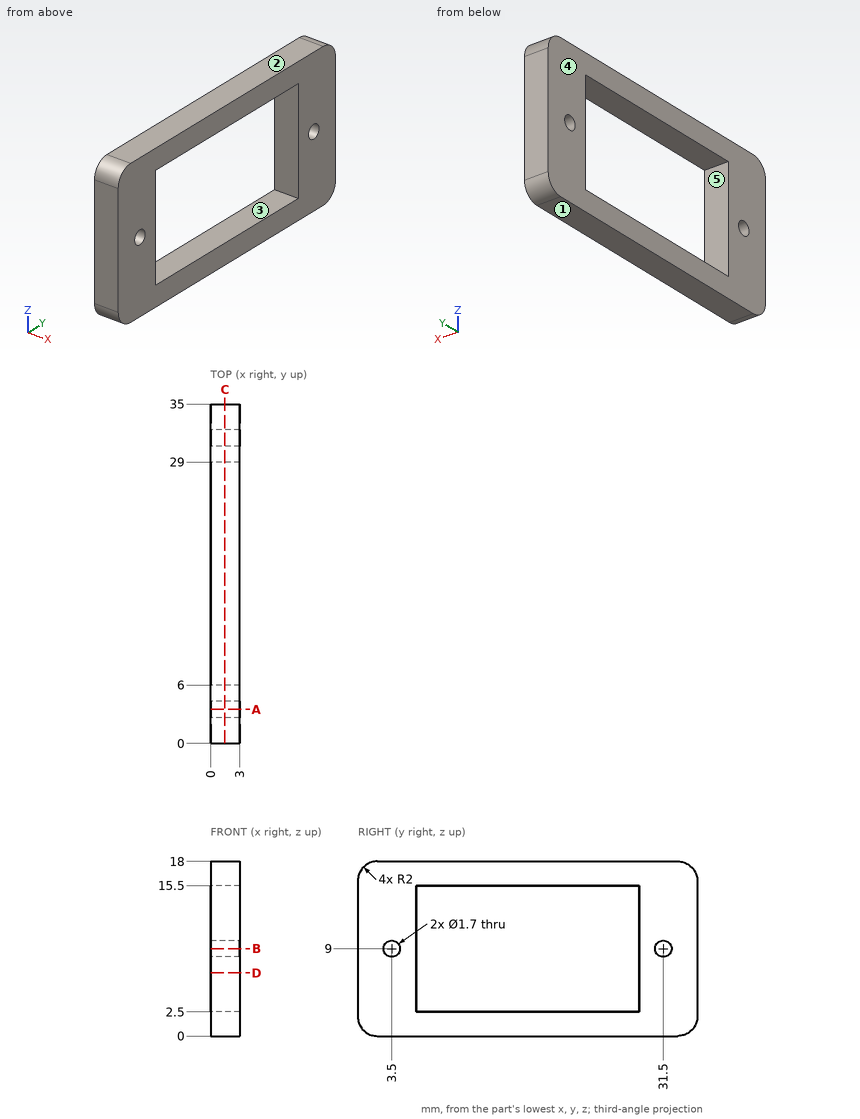
Verification items for this drawing (mm, ordinates from the low corner). A direction names the side the tool comes from. Give positions to 0.01 mm unless a question says otherwise; leave off trailing zeros. Order: outer loops, then holes, each group sorted by start corner. A loop starts at its lowest first (then second) coordinate and runs counter-clockwise, first axis right, second up. Notation, with made-up numbers: M 28.25,-19 L 37.25,-19 A16 cw 37.25,6 Z; hole C 9,-31.5 d11. An arc over 180 degrees is marked long. Use a Markdown table: item, result.
Item 1: Section check B-B (z = 9). Record the cut outline in (x, y).
Answers follow:
| item | result |
|---|---|
| outline | M 0,0 L 3,0 L 3,2.65 L 0,2.65 Z; M 0,4.35 L 3,4.35 L 3,6 L 0,6 Z; M 0,29 L 3,29 L 3,30.65 L 0,30.65 Z; M 0,32.35 L 3,32.35 L 3,35 L 0,35 Z |
Item 2: Draft check along Z on the marked faces 1, 2 and 3. Enter one of: +Z half, -Z half, draft (parallel to the pull), parting line (faces both ways), or undercut.
Answers follow:
| item | result |
|---|---|
| face 1 | -Z half |
| face 2 | +Z half |
| face 3 | undercut |
Item 3: Section check A-A (y = 3.5). Record the cut outline in (x, z), and give its area (3 significant figures).
Answers follow:
| item | result |
|---|---|
| outline | M 0,0 L 3,0 L 3,8.15 L 0,8.15 Z; M 0,9.85 L 3,9.85 L 3,18 L 0,18 Z |
| area | 48.9 mm2 |
Item 4: Section check C-C (x = 1.45). Record the cut outline in (y, z).
Answers follow:
| item | result |
|---|---|
| outline | M 0,2 A2 ccw 2,0 L 33,0 A2 ccw 35,2 L 35,16 A2 ccw 33,18 L 2,18 A2 ccw 0,16 Z; hole C 3.5,9 d1.7; hole M 6,2.5 L 29,2.5 L 29,15.5 L 6,15.5 Z; hole C 31.5,9 d1.7 |
Item 5: Material ranges on line 1 along Y through (x, z) = (0.95, 9); line 2 along Z through (x, y) = (2, 9); line 3 along Y through (x, z) = (1.4, 6.25), recorded low to high.
Answers follow:
| item | result |
|---|---|
| line 1 | y = 0 to 2.65, 4.35 to 6, 29 to 30.65, 32.35 to 35 |
| line 2 | z = 0 to 2.5, 15.5 to 18 |
| line 3 | y = 0 to 6, 29 to 35 |
Item 6: Depth check by flat-ended pin: P1, Ø1.4, axis at y = 31.5, z = 9, coming from the -X side. Enter the tip coordinate at first touch or a pass-through.
Answers follow:
| item | result |
|---|---|
| P1 | passes through |
Item 7: Tool access check on the marked faces 4 and 5. Record the directions out of +Z, -Z, +X, -X, +Y, -Y that give a thin tool (end or side, any length) a straight path to the whole face; none if there is none.
Answers follow:
| item | result |
|---|---|
| face 4 | +Z, -Z, -X, +Y, -Y |
| face 5 | +X, -X |
Item 8: Section check D-D (z = 6.5). Record the cut outline in (x, y), and give its area (3 significant figures).
Answers follow:
| item | result |
|---|---|
| outline | M 0,0 L 3,0 L 3,6 L 0,6 Z; M 0,29 L 3,29 L 3,35 L 0,35 Z |
| area | 36.0 mm2 |
